from build123d import *

# Parameters (mm, degrees)
F0_W     = 50.8
F0_H     = 50.8
F1_DEPTH = 50.8
F2_R     = 15.24
F3_R     = 5.08
F4_DEPTH = 2.54


# Not quite as in the source:
# - a fillet or chamfer that OpenCascade refuses, or shapes differently, is made with other operations: its cross-section is extruded or revolved along the edge and cut away or added


with BuildPart() as f1:
    # F0 (on Top) → F1 (new body)
    with BuildSketch(Plane.XY):
        with Locations((25.4, 25.4)):
            Rectangle(F0_W, F0_H)
    extrude(amount=F1_DEPTH)

    # F2
    f2_edges = [f1.edges().sort_by_distance(p)[0] for p in [
        (50.8, 25.4, 50.8),
        (25.4, 0, 50.8),
        (50.8, 0, 25.4),
        (50.8, 50.8, 25.4),
        (50.8, 25.4, 0),
        (25.4, 0, 0),
        (0, 0, 25.4),
        (0, 25.4, 50.8),
        (25.4, 50.8, 50.8),
        (25.4, 50.8, 0),
        (0, 25.4, 0),
        (0, 50.8, 25.4),
    ]]
    fillet(f2_edges, radius=F2_R)

    # F3 (on face) → F4 (cut)
    with BuildSketch(Plane.XY.offset(50.8)):
        with Locations((25.4, 26.2519493699)):
            Circle(F3_R)
    extrude(amount=-F4_DEPTH, mode=Mode.SUBTRACT)

    # F5: fillet of radius 5.08 on 1 edges, made by hand

    # F5_s1 → F5_t2 (revolve)
    with BuildSketch(Plane.XZ.offset(-26.2519493699)):
        with BuildLine():
            ThreePointArc((30.48, 50.8), (28.6205909488, 48.9405909488), (26.0805909488, 48.26))
            Line((26.0805909488, 48.26), (30.48, 48.26))
            Line((30.48, 48.26), (30.48, 50.8))
        make_face()
    revolve(axis=Axis((25.4, 26.2519493699, 48.26), (0, 0, 1)))


solid = f1.part
The listing builds one solid part. Answer for the finished solid, in the listing's coordinates (mm). Give positions to 0.01 mm unless a question says otherwise; leave off trailing zeros. Write each loop counter-clockwise with the first axis right and the second up, starting at its lowest first coordinate (ties: lowest second). Pieces come first, ordered by that corner, then holes. Notation, with made-up numbers: (82, 7.5) -> (130, 7.5) arc R27 cw to (130, 31.5) -> close; hole circle Ø7 at (37, 89.5). An arc over 180 degrees is marked (long way). Use a Markdown table: item, result.
(1) Determine the mould class of faces 1 (the flat face through (25, 26, 48.26)), 2 (the cylindrical face through (4.35, 25.54, 4.58)), 3 (the flat face through (25, 50.8, 25)), 4 (the cylindrical face through (46.45, 46.22, 25.54)) for opening direction X: released by +X, released by -X, zero draft, split by the parting line, or undercut.
Return value:
| item | result |
|---|---|
| face 1 | undercut |
| face 2 | released by -X |
| face 3 | zero draft |
| face 4 | released by +X |
(2) Section B-B, the plane x = 7 is taken. Determine the outline of the cut face in (y, z).
Return value:
| item | result |
|---|---|
| outline | (2.42, 15.24) arc R12.82 ccw to (15.24, 2.42) -> (35.56, 2.42) arc R12.82 ccw to (48.38, 15.24) -> (48.38, 35.56) arc R12.82 ccw to (35.56, 48.38) -> (15.24, 48.38) arc R12.82 ccw to (2.42, 35.56) -> close |
(3) Flat-ended cylindrical pins translate along their axes: P1, Ø0.7, axis at x = 25.5, y = 26, coming from the +Z side; P2, Ø2, axis at x = 12, z = 30, coming from the +Y side; P3, Ø3, axis at x = 31.5, y = 42.5, coming from the -Z side. Find the tip coordinate at first contact, or state that the pin passes through.
Return value:
| item | result |
|---|---|
| P1 | z = 48.26 |
| P2 | y = 50.63 |
| P3 | z = 1 |
(4) Section A-A, the plane y = 17.5 is taken. Determine the outline of the cut face in (x, z).
Return value:
| item | result |
|---|---|
| outline | (0, 15.24) arc R15.24 ccw to (15.24, 0) -> (35.56, 0) arc R15.24 ccw to (50.8, 15.24) -> (50.8, 35.56) arc R15.24 ccw to (35.56, 50.8) -> (15.24, 50.8) arc R15.24 ccw to (0, 35.56) -> close |
(5) Find the intervals of material crossed by probe 1 along Z at (x, y) = (15, 30); probe 2 along Y at (x, z) = (18, 40.5); probe 3 along X at (y, z) = (20, 42.5), in increasing order. Write a range as from..to.
Return value:
| item | result |
|---|---|
| probe 1 | 0..50.8 |
| probe 2 | 0.82..49.98 |
| probe 3 | 1.67..49.13 |
